Here's how the part is built. I have some questions about the finished solid (model axes, mm). A direction names the side the tool comes from. Coordinates: 2 decimals unless noted, no trailing zeros. Loops run counter-clockwise (first coordinate to the right, second up) from the corner with the lowest first, then second, coordinate; pieces in that order, holes last. Notation, with made-up numbers: (71.5, 84.25) -> (116.5, 84.25) arc R14 cw to (116.5, 106.25) -> close; hole circle Ø6 at (-8.75, 51.25). An arc over 180 degrees is marked (long way). Answer as a JSON object with one key per item and string values. Group by question number.
Q1. Thinking about a two-plate mould opening in X: for faces 4 (the cylindrical face through (4.39, -0.23, 0.74)), 5 (the cylindrical face through (8.823, -0.159, 0.506)), which applies, released by +X, released by -X, zero draft, split by the parting line, or undercut?
Q2. I'm going to push a flat-ended pin straight in: pin 1 (1 mm diameter, centred on x = 3, y = 0.5, fed in from +Z). Where does the tip first touch, or does it pass through?
Q3. On a 3-axis mill with a long thin cutter (end or side, diameter ignored), from which of +Z, -Z, +X, -X, +Y, -Y can I reach the whole of each face in a straight line? I mean faces 1 (the cylindrical face through (3.833, 0.556, -0.726)), 2 (the cylindrical face through (6.247, -0.225, 0.715)), 3 (the cylindrical face through (3.31, 0.43, -0.55)). Say none if no direction works.
Q4. I want a section at C-C on x = 2.75. Write out the boundary of the cut face in (y, z) (1 decimal).
Q5. I need wall thicknesses on line 1 (X direction, y = -0.7, z = 0.55); line 2 (Y direction, x = 7.25, z = -0.25); line 3 (Y direction, x = 2.25, z = 0). Which ranges of each line are inside material? Lowest first, please.
Q6. I want a section at D-D on x = 9.5. Write out the boundary of the cut face in (y, z), then the cut area to 3 significant figures.
```python
from build123d import *


with BuildPart() as part:
    # Sketch1 → Revolve1 (revolve)
    with BuildSketch(Plane.XY, mode=Mode.PRIVATE) as revolve1_sk:
        with BuildLine():
            Line((0, 0), (10.5918, 0))
            ThreePointArc((10.5918, 0), (10.436314706, 0.375374706), (10.06094, 0.53086))
            Line((10.06094, 0.53086), (7.62, 0.53086))
            Line((7.62, 0.53086), (7.62, 0.705305909))
            Line((7.62, 0.705305909), (7.5438, 0.7493))
            Line((7.5438, 0.7493), (4.986785226, 0.7493))
            Line((4.986785226, 0.7493), (4.7498, 0.8128))
            Line((4.7498, 0.8128), (4.7498, 0.7747))
            Line((4.7498, 0.7747), (4.0386, 0.7747))
            Line((4.0386, 0.7747), (4.0386, 0.9144))
            Line((4.0386, 0.9144), (3.6322, 0.9144))
            Line((3.6322, 0.9144), (3.6322, 0.6985))
            Line((3.6322, 0.6985), (2.9972, 0.6985))
            Line((2.9972, 0.6985), (2.921, 0.6223))
            Line((2.921, 0.6223), (2.921, 0.3175))
            Line((2.921, 0.3175), (0.3175, 0.3175))
            ThreePointArc((0.3175, 0.3175), (0.092993597, 0.224506403), (0, 0))
        make_face()
    revolve(revolve1_sk.sketch.rotate(Axis((0, 0, 0), (1, 0, 0)), 90), axis=Axis((0, 0, 0), (1, 0, 0)))


solid = part.part
```
Result set:
{
 "1": {"face 4": "undercut", "face 5": "zero draft"},
 "2": {"pin 1": "stops at z = 0.7"},
 "3": {"face 1": "+X, -X", "face 2": "+X", "face 3": "-X"},
 "4": {"outline": "circle Ø0.6 at (0, 0)"},
 "5": {"line 1": "x = 3.63 to 4.04", "line 2": "y = -0.71 to 0.71", "line 3": "y = -0.32 to 0.32"},
 "6": {"outline": "circle Ø1.06 at (0, 0)", "area": "0.885 mm²"}
}
